```python
from build123d import *

# Parameters (mm, degrees)
SKETCH_1_W               = 71
SKETCH_1_H               = 50
SKETCH_1_R               = 1.05
EXTRUDE_1_DEPTH          = 1.6
SKETCH_2_W               = 6.25
SKETCH_2_H               = 19.25
EXTRUDE_2_DEPTH          = 3.5
EXTRUDE_START            = -1
SKETCH_4_W               = 2
SKETCH_4_H               = 1.5
EXTRUDE_3_DEPTH          = 2.5
CUT_EXTRUDE_1_DEPTH      = 83.071508455
CUT_EXTRUDE_1_DEPTH_BACK = 83.071508455


with BuildPart() as part:
    # Эскиз1 → Бобышка-Вытянуть1 (new body)
    with BuildSketch(Plane.XY):
        with Locations((35.5, 25)):
            Rectangle(SKETCH_1_W, SKETCH_1_H)
        with Locations((2.1, 47.9)):
            Circle(SKETCH_1_R, mode=Mode.SUBTRACT)
        with Locations(Location((68.9, 47.9, 0), (0, 0, 180))):
            Circle(SKETCH_1_R, mode=Mode.SUBTRACT)
        with Locations((68.9, 2.1)):
            Circle(SKETCH_1_R, mode=Mode.SUBTRACT)
        with Locations(Location((2.1, 2.1, 0), (0, 0, 180))):
            Circle(SKETCH_1_R, mode=Mode.SUBTRACT)
    extrude(amount=EXTRUDE_1_DEPTH)

    # Эскиз2 → Бобышка-Вытянуть2 (add)
    with BuildSketch(Plane.XY.offset(1.6)):
        with Locations((40.625, 18.775)):
            Rectangle(SKETCH_2_W, SKETCH_2_H)
    extrude(amount=EXTRUDE_2_DEPTH)

    # Эскиз4 → Бобышка-Вытянуть3 (add)
    with BuildSketch(Plane.XY.offset(5.1).offset(EXTRUDE_START)):
        with Locations((36.5, 27.15)):
            Rectangle(SKETCH_4_W, SKETCH_4_H)
        with Locations((44.75, 27.15)):
            Rectangle(SKETCH_4_W, SKETCH_4_H)
        with Locations((44.75, 24.35)):
            Rectangle(SKETCH_4_W, SKETCH_4_H)
        with Locations((44.75, 21.55)):
            Rectangle(SKETCH_4_W, SKETCH_4_H)
        with Locations((44.75, 18.75)):
            Rectangle(SKETCH_4_W, SKETCH_4_H)
        with Locations((44.75, 15.95)):
            Rectangle(SKETCH_4_W, SKETCH_4_H)
        with Locations((44.75, 13.15)):
            Rectangle(SKETCH_4_W, SKETCH_4_H)
        with Locations((44.75, 10.35)):
            Rectangle(SKETCH_4_W, SKETCH_4_H)
        with Locations((36.5, 24.35)):
            Rectangle(SKETCH_4_W, SKETCH_4_H)
        with Locations((36.5, 21.55)):
            Rectangle(SKETCH_4_W, SKETCH_4_H)
        with Locations((36.5, 18.75)):
            Rectangle(SKETCH_4_W, SKETCH_4_H)
        with Locations((36.5, 15.95)):
            Rectangle(SKETCH_4_W, SKETCH_4_H)
        with Locations((36.5, 13.15)):
            Rectangle(SKETCH_4_W, SKETCH_4_H)
        with Locations((36.5, 10.35)):
            Rectangle(SKETCH_4_W, SKETCH_4_H)
    extrude(amount=-EXTRUDE_3_DEPTH)

    # Эскиз5 → Вырез-Вытянуть1 (cut, two sides: drawn at the far end of the back side and taken through both)
    with BuildSketch(Plane.XZ.offset(-9.15).offset(-CUT_EXTRUDE_1_DEPTH_BACK)):
        Polygon((36, 1.6), (36, 3.716101485), (37.5, 3.716101485), (37.5, 2.1), (43.75, 2.1), (43.75, 3.716101485), (45.25, 3.716101485), (45.25, 1.6), align=None)
    extrude(amount=CUT_EXTRUDE_1_DEPTH + CUT_EXTRUDE_1_DEPTH_BACK, mode=Mode.SUBTRACT)


solid = part.part
```
Can you work these out from the model? Positions are in its coordinate system, mm. A direction names the side the tool comes from. Coordinates: 2 decimals unless noted, no trailing zeros. Loops run counter-clockwise (first coordinate to the right, second up) from the corner with the lowest first, then second, coordinate; pieces in that order, holes last. Notation, with made-up numbers: M 72,47.25 L 130,47.25 A31 ccw 130,82.25 Z; hole C -40,-38 d5. An arc over 180 degrees is marked long. Put each result on its own line as item: value. Start each with the question number.
(1) Which directions (+Z, -Z, +X, -X, +Y, -Y) give clear straight access to the entire face, cutting with the end or side of a thin tool? Please do faces 1 (the face through (45.75, 13, 3)), 2 (the face through (35.8, 12.4, 3)), 3 (the face through (45.41, 13.9, 3.13)), 4 (the face through (36, 10, 3)), 5 (the face through (71, 25, 1)).
(2) Imagine slicing it at C-C on y = 35. List the corners of the cut face in (x, z) for me.
(3) We'd pull the mould along Y, two halves only. Please class faces 6 (the face through (45.25, 24, 3)), 7 (the face through (45.41, 27.9, 3.13)), 8 (the face through (35.8, 9.6, 3)), 9 (the face through (35.8, 18, 3)): +Y half, -Y half, draft (parallel to the pull), parting line (faces both ways), or undercut.
(4) Imagine slicing it at B-B on y = 47.9. List the corners of the cut face in (x, z) for me, and give its area (3 significant figures).
(5) Will these pins go through, and if not, where does the flat tip stop? pin 1 Ø1.2 at (y, z) = (24, 3) entering from +X; pin 2 Ø2 at (x, z) = (36, 3) entering from -Y; pin 3 Ø0.6 at (x, z) = (36, 2.5) entering from +Y.
(6) I need wall thicknesses on probe 1 along Y at (x, z) = (2.1, 0.6); probe 2 along X at (y, z) = (16.5, 2.35); probe 3 along Z at (x, y) = (45.5, 39.5). Which ranges of each line are inside material? Lowest first, please.
(7) Imagine slicing it at A-A on x = 68.9. List the corners of the cut face in (y, z) for me.
(8) Imagine slicing it at D-D on x = 29. List the corners of the cut face in (y, z) for me.
Worked answers:
1. face 1: +Z, +X, +Y, -Y
1. face 2: +Z, -X
1. face 3: +Z, +X
1. face 4: +Y, -Y
1. face 5: +Z, -Z, +X, +Y, -Y
2. outline: M 0,0 L 71,0 L 71,1.6 L 0,1.6 Z
3. face 6: draft
3. face 7: +Y half
3. face 8: -Y half
3. face 9: undercut
4. outline: M 0,0 L 1.05,0 L 1.05,1.6 L 0,1.6 Z; M 3.15,0 L 67.85,0 L 67.85,1.6 L 3.15,1.6 Z; M 69.95,0 L 71,0 L 71,1.6 L 69.95,1.6 Z
4. area: 107 mm2
5. pin 1: stops at x = 45.75
5. pin 2: stops at y = 9.6
5. pin 3: stops at y = 27.9
6. probe 1: y = 0 to 1.05, 3.15 to 46.85, 48.95 to 50
6. probe 2: x = 35.5 to 36, 37.5 to 43.75, 45.25 to 45.75
6. probe 3: z = 0 to 1.6
7. outline: M 0,0 L 1.05,0 L 1.05,1.6 L 0,1.6 Z; M 3.15,0 L 46.85,0 L 46.85,1.6 L 3.15,1.6 Z; M 48.95,0 L 50,0 L 50,1.6 L 48.95,1.6 Z
8. outline: M 0,0 L 50,0 L 50,1.6 L 0,1.6 Z
